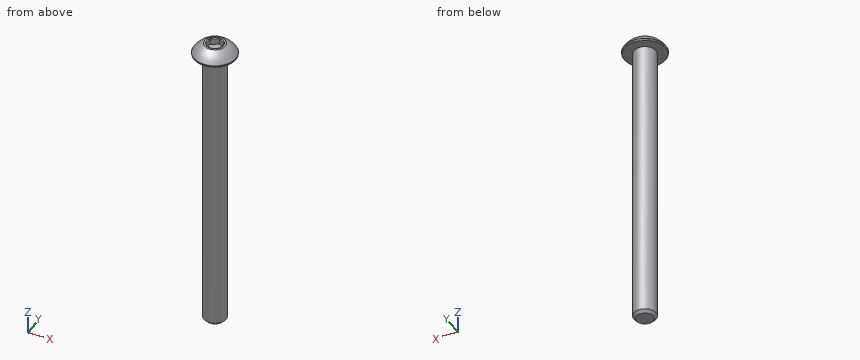
from build123d import *

# Parameters (mm, degrees)
CUT_EXTRUDE1_DEPTH = 1.41097
SKETCH5_R          = 1.833087105
CUT_EXTRUDE2_DEPTH = 1.41097
CUT_EXTRUDE2_DRAFT = -60
FILLET1_R          = 0.12827


with BuildPart() as part:
    # Sketch3 → Revolve1 (revolve)
    with BuildSketch(Plane(origin=(0, 0, 0), x_dir=(0, 0, -1), z_dir=(1, 0, 0))):
        with BuildLine():
            Line((-33.0327, 0), (-33.0327, 2.2225))
            ThreePointArc((-33.0327, 2.2225), (-32.12696038, 3.573966445), (-30.85211, 4.5847))
            Line((-30.85211, 4.5847), (-30.4673, 4.516847615))
            Line((-30.4673, 4.516847615), (-30.4673, 2.413))
            Line((-30.4673, 2.413), (32.4373875, 2.413))
            Line((32.4373875, 2.413), (33.0327, 1.8176875))
            Line((33.0327, 1.8176875), (33.0327, 0))
            Line((33.0327, 0), (-33.0327, 0))
        make_face()
    revolve(axis=Axis((0, 0, 33.0327), (0, 0, -1)))

    # Sketch4 → Cut-Extrude1 (cut)
    with BuildSketch(Plane.XY.offset(33.0327)):
        Polygon((-1.5875, -0.916543552), (0, -1.833087105), (1.5875, -0.916543552), (1.5875, 0.916543552), (0, 1.833087105), (-1.5875, 0.916543552), align=None)
    extrude(amount=-CUT_EXTRUDE1_DEPTH, mode=Mode.SUBTRACT)


with BuildPart() as cut_extrude2_tool:
    # Sketch5 → Cut-Extrude2 (with draft: the straight prism first)
    with BuildSketch(Plane.XY.offset(33.0327)):
        Circle(SKETCH5_R)
    extrude(amount=-CUT_EXTRUDE2_DEPTH)
    # Cut-Extrude2: the draft: its side faces are tilted about the plane it starts from
    cut_extrude2_sides = [cut_extrude2_tool.faces().sort_by_distance(p)[0] for p in [
        (-1.833087105, 0, 32.327215),
    ]]
    draft(cut_extrude2_sides, Plane.XY.offset(33.0327), CUT_EXTRUDE2_DRAFT)


with BuildPart() as part_1:
    add(part.part)

    # Cut-Extrude2: cut by cut_extrude2_tool
    add(cut_extrude2_tool.part, mode=Mode.SUBTRACT)

    # Fillet1
    fillet1_edges = [part_1.edges().sort_by_distance(p)[0] for p in [
        (0, -4.516847615, 30.4673),
        (0, -4.5847, 30.85211),
    ]]
    fillet(fillet1_edges, radius=FILLET1_R)


solid = part_1.part
The listing builds one solid part. Answer for the finished solid, in the listing's coordinates (mm). Round coordinates to 2 decimals unless told otherwise and drop trailing zeros. Loops run counter-clockwise (first coordinate to the right, second up) from the corner with the lowest first, then second, coordinate; pieces in that order, holes last. Notation, with made-up numbers: M 35.5,0.25 L 40.5,0.25 A27 cw 40.5,35.25 Z; hole C -11.75,-14.5 d11. An arc over 180 degrees is marked long. Return JSON: item names as keys, results as strings.
Q1. Each of these flat-tipped pins is pushed along its axis until it touches: pin 1 Ø5 at (x, z) = (-3.5, 9.5) entering from +Y; pin 2 Ø1 at (x, y) = (1.5, 3.5) entering from +Z; pin 3 Ø3 at (y, z) = (2, -19) entering from +X. Where does it stop, or does it pass through?
Results list:
{"pin 1": "stops at y = 2.2", "pin 2": "stops at z = 32.36", "pin 3": "stops at x = 2.36"}
Q2. Find the intervals of material crossed by line 1 along X through (y, z) = (-0.25, -14.5); line 2 along X through (y, z) = (-2, -20); line 3 along Y through (x, z) = (0.5, -29), in increasing order. Write a range as from..to.
Results list:
{"line 1": "x = -2.4..2.4", "line 2": "x = -1.35..1.35", "line 3": "y = -2.36..2.36"}
Q3. Find section A-A, the plane z = 3.5. Determine the outline of the cut face in (x, y).
Results list:
{"outline": "C 0,0 d4.83"}
